Read the model definition and answer for the solid it produces. Units are mm, in the model's axes. A direction names the side the tool comes from. Round coordinates to 2 decimals unless told otherwise and drop trailing zeros. Order: outer loops, then holes, each group sorted by start corner. A loop starts at its lowest first (then second) coordinate and runs counter-clockwise, first axis right, second up. Notation, with made-up numbers: (53.25, -25.75) - (89.25, -25.75) arc R15 ccw to (89.25, -13.75) - close; hole circle Ø6 at (-10.5, 63). An arc over 180 degrees is marked (long way). Answer as a JSON object with one key per item and string values. Group by question number.
Q1. The mould has two halves that part along Y. Classify faces 3 (the flat face through (8.67, -6.16, 2.54)), 4 (the cylindrical face through (-26.35, -5.67, 2.54)), 5 (the flat face through (-10, -2, 5)): pulls with the +Y half, pulls with the -Y half, needs draft (parallel to the pull), parting line crosses it, or undercut.
Q2. Given pin 1 Ø2 at (x, z) = (5, 0.5) entering from +Y; pin 2 Ø1.5 at (x, z) = (6.5, 1.5) entering from -Y; pin 3 Ø3 at (x, z) = (-6.5, 1) entering from +Y, each flat-ended and moving along its own axis, determine where each tip first touches the part or whether it passes through.
Q3. A cutting plane is placed at B-B on x = -4. Determine the outline of the cut face in (y, z).
Q4. A cutting plane is placed at A-A on y = 12. Determine the outline of the cut face in (x, z).
Q5. A tool of negligible diameter and unlimited length cuts with its end or side. For faces 1 (the cylindrical face through (-2.616, 10.338, 2.465)), 2 (the flat face through (4.16, 10.67, 2.54)), from which of +Z, -Z, +X, -X, +Y, -Y can it reach the whole face along a straight path? Write none if from no direction.
Q6. Consider line 1 (Y direction, x = 3, z = 0.4); line 2 (Y direction, x = -4, z = 2.6); line 3 (X direction, y = 11.5, z = 4.15). Determine where each line is inside the solid, lowest interval first.
Q7. A cutting plane is placed at C-C on z = 2.1. Determine the outline of the cut face in (x, y), and give its area (3 significant figures).
Q8. A cutting plane is placed at D-D on x = -19.5. Determine the outline of the cut face in (y, z).
```python
from build123d import *

# Parameters (mm, degrees)
CYLINDER001_R            = 3
CYLINDER001_DEPTH        = 5
CYLINDER_W               = 25
CYLINDER_H               = 5
CYLINDER_ANGLE           = 270
CYLINDER_PLACEMENT_ANGLE = 60


with BuildPart() as cilindro001:
    # Cylinder001 → Cylinder001 (new body)
    with BuildSketch(Plane(origin=(-4, 13, 0), x_dir=(1, 0, 0), z_dir=(0, 0, 1))):
        Circle(CYLINDER001_R)
    extrude(amount=CYLINDER001_DEPTH)


with BuildPart() as obj1:
    # Cylinder → Cylinder (revolve)
    with BuildSketch(Plane.XZ):
        with Locations((12.5, 2.5)):
            Rectangle(CYLINDER_W, CYLINDER_H)
    revolve(axis=Axis((0, 0, 0), (0, 0, 1)), revolution_arc=CYLINDER_ANGLE)


with BuildPart() as obj1_1:
    # Cylinder placement: moved
    add(obj1.part.moved(Location((-2, 0, 0))).rotate(Axis((-2, 0, 0), (0, 0, 1)), CYLINDER_PLACEMENT_ANGLE))

    # Cut: cut Cilindro001
    add(cilindro001.part, mode=Mode.SUBTRACT)


solid = obj1_1.part
```
Result set:
{
 "1": {"face 3": "undercut", "face 4": "parting line crosses it", "face 5": "needs draft"},
 "2": {"pin 1": "stops at y = 24.27", "pin 2": "stops at y = -23.77", "pin 3": "stops at y = 24.82"},
 "3": {"outline": "(-24.92, 0) - (10, 0) - (10, 5) - (-24.92, 5) - close; (16, 0) - (24.92, 0) - (24.92, 5) - (16, 5) - close"},
 "4": {"outline": "(-23.93, 0) - (-6.83, 0) - (-6.83, 5) - (-23.93, 5) - close; (-1.17, 0) - (4.93, 0) - (4.93, 5) - (-1.17, 5) - close"},
 "5": {"face 1": "+Z, -Z", "face 2": "+Z, -Z, +X"},
 "6": {"line 1": "y = -24.49 to -2.89, 8.66 to 24.49", "line 2": "y = -24.92 to 10, 16 to 24.92", "line 3": "x = -24.2 to -6.6, -1.4 to 4.64"},
 "7": {"outline": "(-2, 0) - (10.5, 21.65) arc R25 ccw (long way) to (19.65, -12.5) - close; hole circle Ø6 at (-4, 13)", "area": "1,440 mm²"},
 "8": {"outline": "(-17.85, 0) - (17.85, 0) - (17.85, 5) - (-17.85, 5) - close"}
}
